Read the model definition and answer for the solid it produces. Units are mm, in the model's axes. A direction names the side the tool comes from. Coordinates: 2 decimals unless noted, no trailing zeros. Order: outer loops, then holes, each group sorted by start corner. A loop starts at its lowest first (then second) coordinate and runs counter-clockwise, first axis right, second up. Notation, with made-up numbers: (8.5, -35) - (50.5, -35) arc R24 ccw to (50.5, 1) - close; hole circle Ø7 at (59.5, -39.75). An arc over 180 degrees is marked (long way). Write item = value, one per line.
from build123d import *

# Parameters (mm, degrees)
SKETCH2_W           = 175
SKETCH2_H           = 90
SKETCH2_W_2         = 155
SKETCH2_H_2         = 60
BOSS_EXTRUDE3_DEPTH = 52.5
SKETCH3_R           = 6
SKETCH3_R_2         = 15
CUT_EXTRUDE1_DEPTH  = 80
SKETCH4_W           = 175
SKETCH4_H           = 12.5
CUT_EXTRUDE2_DEPTH  = 10


with BuildPart() as part:
    # Sketch2 → Boss-Extrude3 (new, symmetric)
    with BuildSketch(Plane(origin=(0, 0, 0), x_dir=(1, 0, 0), z_dir=(0, 1, 0))):
        with Locations((0, 45)):
            Rectangle(SKETCH2_W, SKETCH2_H)
        with Locations((0, 50)):
            Rectangle(SKETCH2_W_2, SKETCH2_H_2, mode=Mode.SUBTRACT)
    extrude(amount=BOSS_EXTRUDE3_DEPTH, both=True)

    # Sketch3 → Cut-Extrude1 (cut)
    with BuildSketch(Plane.XY):
        with BuildLine():
            Line((-87.5, 52.5), (-87.5, 40))
            Line((-87.5, 40), (-34.003676272, 40))
            ThreePointArc((-34.003676272, 40), (-18.114220897, 49.276008374), (7.6e-08, 52.5))
            Line((7.6e-08, 52.5), (-87.5, 52.5))
        make_face()
        with BuildLine():
            Line((87.5, 52.5), (7.6e-08, 52.5))
            ThreePointArc((7.6e-08, 52.5), (18.114220968, 49.276008348), (34.003676272, 40))
            Line((34.003676272, 40), (87.5, 40))
            Line((87.5, 40), (87.5, 52.5))
        make_face()
        with BuildLine():
            Line((-34.003676272, -40), (-87.5, -40))
            Line((-87.5, -40), (-87.5, -52.5))
            Line((-87.5, -52.5), (0, -52.5))
            ThreePointArc((0, -52.5), (-18.114220933, -49.276008361), (-34.003676272, -40))
        make_face()
        with BuildLine():
            ThreePointArc((34.003676272, -40), (18.114220933, -49.276008361), (0, -52.5))
            Line((0, -52.5), (87.5, -52.5))
            Line((87.5, -52.5), (87.5, -40))
            Line((87.5, -40), (34.003676272, -40))
        make_face()
        with BuildLine():
            Line((87.5, 30), (43.084219849, 30))
            ThreePointArc((43.084219849, 30), (50.090775309, 15.721457597), (52.5, 0))
            ThreePointArc((52.5, 0), (50.090775309, -15.721457597), (43.084219849, -30))
            Line((43.084219849, -30), (87.5, -30))
            Line((87.5, -30), (87.5, 30))
        make_face()
        with BuildLine():
            Line((-43.084219849, 30), (-87.5, 30))
            Line((-87.5, 30), (-87.5, -30))
            Line((-87.5, -30), (-43.084219849, -30))
            ThreePointArc((-43.084219849, -30), (-52.5, 0), (-43.084219849, 30))
        make_face()
        with Locations((-8.900837358, 38.997116487)):
            Circle(SKETCH3_R)
        with Locations((24.939592074, 31.273259299)):
            Circle(SKETCH3_R)
        with Locations((-36.038754716, 17.355349565)):
            Circle(SKETCH3_R)
        with Locations((40, 0)):
            Circle(SKETCH3_R)
        with Locations((-36.038754716, -17.355349565)):
            Circle(SKETCH3_R)
        with Locations((-8.900837358, -38.997116487)):
            Circle(SKETCH3_R)
        with Locations((24.939592074, -31.273259299)):
            Circle(SKETCH3_R)
        Circle(SKETCH3_R_2)
    extrude(amount=-CUT_EXTRUDE1_DEPTH, mode=Mode.SUBTRACT)

    # Sketch4 → Cut-Extrude2 (cut)
    with BuildSketch(Plane.XY.offset(-80)):
        with Locations((0, 46.25)):
            Rectangle(SKETCH4_W, SKETCH4_H)
        with Locations((0, -46.25)):
            Rectangle(SKETCH4_W, SKETCH4_H)
    extrude(amount=-CUT_EXTRUDE2_DEPTH, mode=Mode.SUBTRACT)


solid = part.part
1) Flat-ended cylindrical pins translate along their axes: pin 1 Ø22 at (x, z) = (76, -45) entering from +Y; pin 2 Ø3 at (x, y) = (-64, 13.5) entering from +Z. Find the tip coordinate at first contact, or state that the pin passes through.
Returned:
pin_1 = 40
pin_2 = -80
2) The part is cut by section D-D (z = -4.5). Count the separate pieces of the cut face and the enclosed holes in it, and give its area (3 significant figures).
Returned:
separate_pieces = 1
enclosed_holes = 8
area = 9,100 mm^2
3) The part is cut by section A-A (z = -71). Determine the outline of the cut face in (x, y).
Returned:
outline = (-87.5, -40) - (-77.5, -40) - (-77.5, -30) - (-87.5, -30) - close; (-87.5, 30) - (-77.5, 30) - (-77.5, 40) - (-87.5, 40) - close; (77.5, -40) - (87.5, -40) - (87.5, -30) - (77.5, -30) - close; (77.5, 30) - (87.5, 30) - (87.5, 40) - (77.5, 40) - close
4) Determine the mould class of faces 1 (the face through (-80, -30, -22)), 2 (the face through (-30.496, -19.653, -9.86)), 3 (the face through (34, 0, -10)), 4 (the face through (-87.5, -3, -81)) for opening direction X: pulls with the +X half, pulls with the -X half, needs draft (parallel to the pull), parting line crosses it, or undercut.
Returned:
face_1 = needs draft
face_2 = undercut
face_3 = undercut
face_4 = pulls with the -X half
5) Straight lines are drawn through the part: line 1 along Y through (x, z) = (-43.5, -4.5); line 2 along Y through (x, z) = (79.5, -49); line 3 along Z through (x, y) = (36, -37.5). For each, find the intervals that lie inside material, in ascending order. Write a range as from..to.
Returned:
line_1 = -40..-30, -29.39..29.39, 30..40
line_2 = -40..-30, 30..40
line_3 = -90..-80, -20..0
6) The part is cut by section C-C (y = 27.5). Determine the outline of the cut face in (x, z).
Returned:
outline = (-87.5, -90) - (87.5, -90) - (87.5, -80) - (-87.5, -80) - close; (-44.72, -20) - (20.27, -20) - (20.27, 0) - (-44.72, 0) - close; (29.6, -20) - (44.72, -20) - (44.72, 0) - (29.6, 0) - close
7) For faces 5 (the face through (77.5, -35, -50)), 6 (the face through (-20, 40, -81)), 7 (the face through (-9.682, -33.048, -9.86)), 8 (the face through (-21, 1, 0)), 9 (the face through (-80, 30, -22)), determine the directions among +Z, -Z, +X, -X, +Y, -Y from which every point of the face is accessible in a straight line to the end or side of a thin tool.
Returned:
face_5 = +Y, -Y
face_6 = -Z, +Y
face_7 = +Z
face_8 = +Z, +X, -X, +Y, -Y
face_9 = +Z, -X
8) The part is cut by section B-B (x = 40). Determine the outline of the cut face in (y, z).
Returned:
outline = (-40, -90) - (40, -90) - (40, -80) - (-40, -80) - close; (-40, -20) - (-6, -20) - (-6, 0) - (-40, 0) - close; (6, -20) - (40, -20) - (40, 0) - (6, 0) - close
